```python
from build123d import *

# Parameters (mm, degrees)
SKETCH1_W              = 72
SKETCH1_H              = 47
BOSS_EXTRUDE1_DEPTH    = 1.6
SKETCH2_W              = 20
SKETCH2_H              = 3
BOSS_EXTRUDE2_DEPTH    = 2.6
SKETCH3_W              = 45
SKETCH3_H              = 45
SKETCH3_R              = 1.325
BOSS_EXTRUDE3_DEPTH    = 1.05
SKETCH4_W              = 40
SKETCH4_H              = 34
BOSS_EXTRUDE4_DEPTH    = 3.9
CUT_EXTRUDE1_DEPTH     = 0.1
FILLET1_R              = 1
SKETCH6_W              = 12
SKETCH6_H              = 12
BOSS_EXTRUDE5_DEPTH    = 3.65
SKETCH7_R              = 3.5
BOSS_EXTRUDE6_DEPTH    = 0.2
SKETCH8_W              = 2.9
SKETCH8_H              = 2.9
BOSS_EXTRUDE7_DEPTH    = 1.2
SKETCH9_W              = 3.7
SKETCH9_H              = 3.7
BOSS_EXTRUDE8_DEPTH    = 2.3
FILLET2_R              = 0.5
SKETCH10_R             = 1
CUT_EXTRUDE2_DEPTH     = 3
LPATTERN1_COUNT        = 3
LPATTERN1_PITCH        = 15.24
FILLET2_OF_LPATTERN1_R = 0.5


with BuildPart() as part:
    # Sketch1 → Boss-Extrude1 (new body)
    with BuildSketch(Plane(origin=(0, 0, 0), x_dir=(1, 0, 0), z_dir=(0, 1, 0))):
        Rectangle(SKETCH1_W, SKETCH1_H)
    extrude(amount=BOSS_EXTRUDE1_DEPTH)

    # Sketch2 → Boss-Extrude2 (add)
    with BuildSketch(Plane(origin=(0, 1.6, 0), x_dir=(1, 0, 0), z_dir=(0, 1, 0))):
        with Locations((-19, -19.975114796)):
            Rectangle(SKETCH2_W, SKETCH2_H)
        with Locations((-19, 19.975114796)):
            Rectangle(SKETCH2_W, SKETCH2_H)
    extrude(amount=BOSS_EXTRUDE2_DEPTH)

    # Sketch3 → Boss-Extrude3 (add)
    with BuildSketch(Plane(origin=(0, 4.2, 0), x_dir=(1, 0, 0), z_dir=(0, 1, 0))):
        with Locations((-19.35, -0.35)):
            Rectangle(SKETCH3_W, SKETCH3_H)
        with Locations((-39.35, 19.65)):
            Circle(SKETCH3_R, mode=Mode.SUBTRACT)
        with Locations((0.65, 19.65)):
            Circle(SKETCH3_R, mode=Mode.SUBTRACT)
        with Locations((0.65, -20.35)):
            Circle(SKETCH3_R, mode=Mode.SUBTRACT)
        with Locations((-39.35, -20.35)):
            Circle(SKETCH3_R, mode=Mode.SUBTRACT)
    extrude(amount=BOSS_EXTRUDE3_DEPTH)

    # Sketch4 → Boss-Extrude4 (add)
    with BuildSketch(Plane(origin=(0, 5.25, 0), x_dir=(1, 0, 0), z_dir=(0, 1, 0))):
        with Locations((-19.25, -0.25)):
            Rectangle(SKETCH4_W, SKETCH4_H)
    extrude(amount=BOSS_EXTRUDE4_DEPTH)

    # Sketch5 → Cut-Extrude1 (cut)
    with BuildSketch(Plane(origin=(0, 9.15, 0), x_dir=(1, 0, 0), z_dir=(0, 1, 0))):
        with BuildLine():
            Line((-34.55, -15.8), (-3.95, -15.8))
            ThreePointArc((-3.95, -15.8), (-1.828679656, -14.921320344), (-0.95, -12.8))
            Line((-0.95, -12.8), (-0.95, 7.5))
            ThreePointArc((-0.95, 7.5), (-1.828679656, 9.621320344), (-3.95, 10.5))
            Line((-3.95, 10.5), (-34.55, 10.5))
            ThreePointArc((-34.55, 10.5), (-36.671320344, 9.621320344), (-37.55, 7.5))
            Line((-37.55, 7.5), (-37.55, -12.8))
            ThreePointArc((-37.55, -12.8), (-36.671320344, -14.921320344), (-34.55, -15.8))
        make_face()
    extrude(amount=-CUT_EXTRUDE1_DEPTH, mode=Mode.SUBTRACT)

    # Fillet1
    fillet1_edges = [part.edges().sort_by_distance(p)[0] for p in [
        (-39.25, 7.2, -16.75),
        (-39.25, 7.2, 17.25),
        (0.75, 7.2, 17.25),
        (0.75, 7.2, -16.75),
    ]]
    fillet(fillet1_edges, radius=FILLET1_R)

    # Sketch6 → Boss-Extrude5 (add)
    with BuildSketch(Plane(origin=(0, 1.6, 0), x_dir=(1, 0, 0), z_dir=(0, 1, 0))):
        with Locations((11.35, -15.05)):
            Rectangle(SKETCH6_W, SKETCH6_H)
    boss_extrude5 = extrude(amount=BOSS_EXTRUDE5_DEPTH)

    # Sketch7 → Boss-Extrude6 (add)
    with BuildSketch(Plane(origin=(0, 5.25, 0), x_dir=(1, 0, 0), z_dir=(0, 1, 0))):
        with Locations((11.35, -15.05)):
            Circle(SKETCH7_R)
    boss_extrude6 = extrude(amount=BOSS_EXTRUDE6_DEPTH)

    # Sketch8 → Boss-Extrude7 (add)
    with BuildSketch(Plane(origin=(0, 5.45, 0), x_dir=(1, 0, 0), z_dir=(0, 1, 0))):
        with Locations((11.35, -15.05)):
            Rectangle(SKETCH8_W, SKETCH8_H)
    boss_extrude7 = extrude(amount=BOSS_EXTRUDE7_DEPTH)

    # Sketch9 → Boss-Extrude8 (add)
    with BuildSketch(Plane(origin=(0, 6.65, 0), x_dir=(1, 0, 0), z_dir=(0, 1, 0))):
        with Locations((11.35, -15.05)):
            Rectangle(SKETCH9_W, SKETCH9_H)
    boss_extrude8 = extrude(amount=BOSS_EXTRUDE8_DEPTH)

    # Fillet2
    fillet2_edges = [part.edges().sort_by_distance(p)[0] for p in [
        (5.35, 3.425, 9.05),
        (5.35, 3.425, 21.05),
        (17.35, 3.425, 21.05),
        (17.35, 3.425, 9.05),
        (9.5, 7.8, 13.2),
        (9.5, 7.8, 16.9),
        (13.2, 7.8, 16.9),
        (13.2, 7.8, 13.2),
    ]]
    fillet(fillet2_edges, radius=FILLET2_R)

    # Sketch10 → Cut-Extrude2 (cut)
    with BuildSketch(Plane(origin=(0, 8.95, 0), x_dir=(1, 0, 0), z_dir=(0, 1, 0))):
        with Locations((11.35, -15.05)):
            Circle(SKETCH10_R)
    cut_extrude2 = extrude(amount=-CUT_EXTRUDE2_DEPTH, mode=Mode.SUBTRACT)

    # LPattern1: Boss-Extrude5, Boss-Extrude6, Boss-Extrude7, Boss-Extrude8, Cut-Extrude2 ×3
    with Locations(*[(0, 0, -i * LPATTERN1_PITCH) for i in range(1, LPATTERN1_COUNT)]):
        add(boss_extrude5)
        add(boss_extrude6)
        add(boss_extrude7)
        add(boss_extrude8)
        add(cut_extrude2, mode=Mode.SUBTRACT)

    # Fillet2 of LPattern1
    fillet2_of_lpattern1_edges = [part.edges().sort_by_distance(p)[0] for p in [
        (5.35, 3.425, -6.19),
        (5.35, 3.425, 5.81),
        (17.35, 3.425, 5.81),
        (17.35, 3.425, -6.19),
        (9.5, 7.8, -2.04),
        (9.5, 7.8, 1.66),
        (13.2, 7.8, 1.66),
        (13.2, 7.8, -2.04),
        (5.35, 3.425, -21.43),
        (5.35, 3.425, -9.43),
        (17.35, 3.425, -9.43),
        (17.35, 3.425, -21.43),
        (9.5, 7.8, -17.28),
        (9.5, 7.8, -13.58),
        (13.2, 7.8, -13.58),
        (13.2, 7.8, -17.28),
    ]]
    fillet(fillet2_of_lpattern1_edges, radius=FILLET2_OF_LPATTERN1_R)


solid = part.part
```
Geometry check sheet. Reference: the model listing, model coordinates, mm. A direction names the side the tool comes from. Coordinates: 2 decimals unless noted, no trailing zeros. Order: outer loops, then holes, each group sorted by start corner. A loop starts at its lowest first (then second) coordinate and runs counter-clockwise, first axis right, second up.
Q1. Sectioned sample at A-A on x = -31.5. Record the cut outline in (y, z).
Reply:
outline: (0, -23.5) - (1.6, -23.5) - (1.6, 23.5) - (0, 23.5) - close; (4.2, -22.15) - (5.25, -22.15) - (5.25, -16.75) - (9.15, -16.75) - (9.15, -10.5) - (9.05, -10.5) - (9.05, 15.8) - (9.15, 15.8) - (9.15, 17.25) - (5.25, 17.25) - (5.25, 22.85) - (4.2, 22.85) - close
Q2. Depth check by flat-ended pin: pin 1 Ø1.3 at (x, y) = (-16, 2.5) entering from +Z; pin 2 Ø4 at (y, z) = (5, 9) entering from +X; pin 3 Ø1 at (x, y) = (11, 6) entering from +Z; pin 4 Ø3 at (x, z) = (12, 16) entering from -Y. Enter the tip coordinate at first touch or a pass-through.
Reply:
pin 1: stops at z = 21.48
pin 2: stops at x = 17.35
pin 3: stops at z = 16.5
pin 4: stops at y = 0
Q3. Sectioned sample at B-B on y = 8. Give the number of separate pieces and of enclosed holes in the cut face, and give its area (3 significant figures).
Reply:
separate pieces: 4
enclosed holes: 3
area: 1,390 mm2
Q4. Sectioned sample at C-C on z = -8.5. Record the cut outline in (x, y), and give its area (3 significant figures).
Reply:
outline: (-41.85, 4.2) - (3.15, 4.2) - (3.15, 5.25) - (0.75, 5.25) - (0.75, 9.15) - (-1.12, 9.15) - (-1.12, 9.05) - (-37.38, 9.05) - (-37.38, 9.15) - (-39.25, 9.15) - (-39.25, 5.25) - (-41.85, 5.25) - close; (-36, 0) - (36, 0) - (36, 1.6) - (-36, 1.6) - close
area: 315 mm2
Q5. Thickness scan on probe 1 along X at (y, z) = (7.9, 15.05); probe 2 along Z at (x, y) = (11.35, 7.35); probe 3 along Z at (x, y) = (0.65, 4.85) (3 decimals). Record the ranges inside material, lowest first.
Reply:
probe 1: x = -39.25 to 0.75, 9.5 to 10.35, 12.35 to 13.2
probe 2: z = -17.28 to -16.43, -14.43 to -13.58, -2.04 to -1.19, 0.81 to 1.66, 13.2 to 14.05, 16.05 to 16.9
probe 3: z = -22.15 to -20.975, -18.325 to 19.025, 21.675 to 22.85
Q6. Draft check along Y on faces 6 (the face through (11, 5.95, 0)), 7 (the face through (11.81, 7.47, 15.94)), 8 (the face through (11.3, 6.65, -13.8)). Enter one of: released by +Y, released by -Y, zero draft, split by the parting line, or undercut.
Reply:
face 6: released by +Y
face 7: zero draft
face 8: undercut
Q7. Tool access check on faces 1 (the face through (5.35, 3, 0)), 2 (the face through (-9, 3, -20)), 3 (the face through (11, 3, 5.81)), 4 (the face through (17.35, 3, 0)), 5 (the face through (-19, 3, -18.475)). Record the directions out of +Z, -Z, +X, -X, +Y, -Y that give a thin tool (end or side, any length) a straight path to the whole face; none if there is none.
Reply:
face 1: +Z, -Z, +Y
face 2: +Z, -Z
face 3: +X, +Y
face 4: +Z, -Z, +X, +Y
face 5: -X
